Design review of the part shown in the three views and the two pictorial views. Dimensions are in mm from the part's minimum x, y and z. Round coordinates to 2 decimals unless told otherwise and drop trailing zeros. Loops run counter-clockwise (first coordinate to the right, second up) from the corner with the lowest first, then second, coordinate; pieces in that order, holes last.
1) Take a section at A-A (y = 21.15). State the section outline as (x, z) points, then the cut area to 3 significant figures.
2) Take a section at B-B (z = 1.7). State the section outline as (x, y) points, then the cut area to 3 significant figures.
3) Take a section at D-D (y = 5.65). State the section outline as (x, z) points.
4) Wall thickness on L1, parallel to Y at x = 21.15, z = 1.1; L2, parallel to X at y = 5.65, z = 1.2; L3, parallel to Y at x = 22, z = 2.5: over which ranges is each line inside the solid? List them lowest first.
5) Take a section at C-C (x = 5.65). State the section outline as (y, z) points.
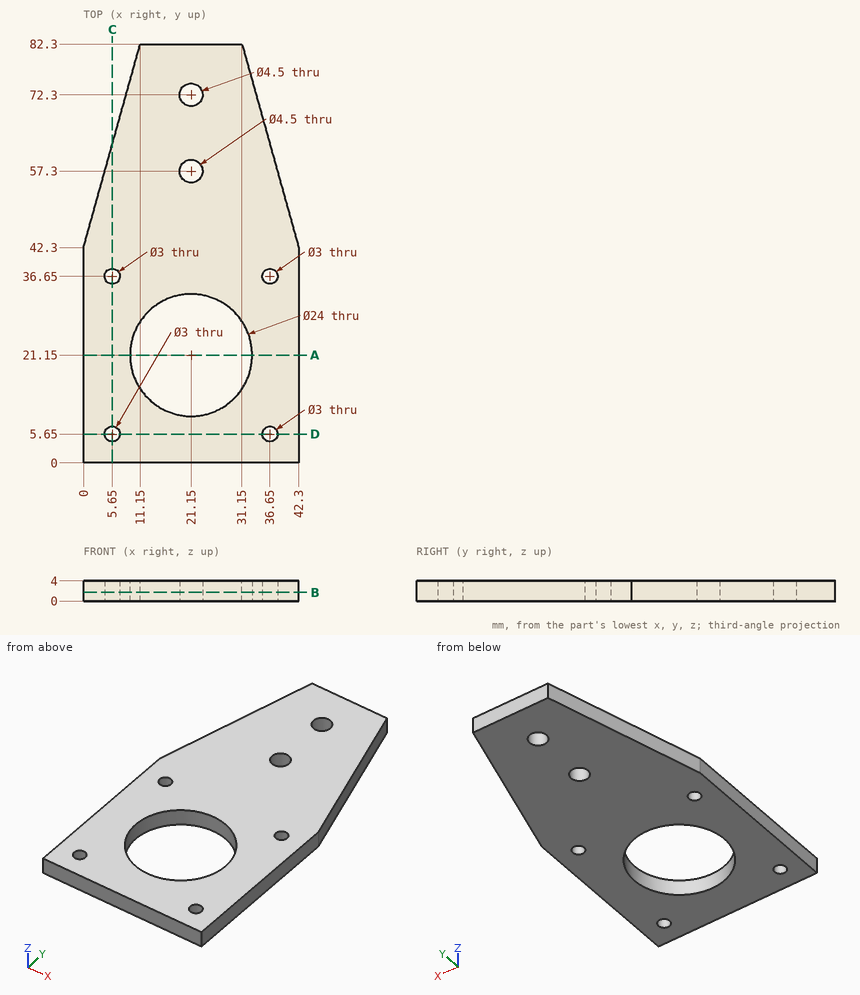
Response:
1. outline: (0, 0) - (9.15, 0) - (9.15, 4) - (0, 4) - close; (33.15, 0) - (42.3, 0) - (42.3, 4) - (33.15, 4) - close
1. area: 73.2 mm2
2. outline: (0, 0) - (42.3, 0) - (42.3, 42.3) - (31.15, 82.3) - (11.15, 82.3) - (0, 42.3) - close; hole circle Ø3 at (5.65, 5.65); hole circle Ø3 at (5.65, 36.65); hole circle Ø24 at (21.15, 21.15); hole circle Ø4.5 at (21.15, 57.3); hole circle Ø4.5 at (21.15, 72.3); hole circle Ø3 at (36.65, 5.65); hole circle Ø3 at (36.65, 36.65)
2. area: 2,520 mm2
3. outline: (0, 0) - (4.15, 0) - (4.15, 4) - (0, 4) - close; (7.15, 0) - (35.15, 0) - (35.15, 4) - (7.15, 4) - close; (38.15, 0) - (42.3, 0) - (42.3, 4) - (38.15, 4) - close
4. L1: y = 0 to 9.15, 33.15 to 55.05, 59.55 to 70.05, 74.55 to 82.3
4. L2: x = 0 to 4.15, 7.15 to 35.15, 38.15 to 42.3
4. L3: y = 0 to 9.18, 33.12 to 55.22, 59.38 to 70.22, 74.38 to 82.3
5. outline: (0, 0) - (4.15, 0) - (4.15, 4) - (0, 4) - close; (7.15, 0) - (35.15, 0) - (35.15, 4) - (7.15, 4) - close; (38.15, 0) - (62.57, 0) - (62.57, 4) - (38.15, 4) - close
